Design review of the part built by this model. Coordinates are the model's own, in mm. A direction names the side the tool comes from. Round coordinates to 2 decimals unless told otherwise and drop trailing zeros. Loops run counter-clockwise (first coordinate to the right, second up) from the corner with the lowest first, then second, coordinate; pieces in that order, holes last. Notation, with made-up numbers: (85, 40.25) -> (126, 40.25) arc R17 ccw to (126, 52.25) -> close; hole circle Ø10 at (0, 55.25). An arc over 180 degrees is marked (long way). Answer as CSV lines item,"result". Start each with the question number.
```python
from build123d import *

# Parameters (mm, degrees)
F0_R     = 6.35
F1_DEPTH = 12.7


with BuildPart() as f1:
    # F0 (on Top) → F1 (new body)
    with BuildSketch(Plane.XY):
        Polygon((-7.92159, -12.359408), (-7.92159, -30.139408), (-33.32159, -30.139408), (-38.40159, -55.026224), (-7.92159, -55.026224), (-7.92159, -72.806224), (30.17841, -72.806224), (30.17841, -55.026224), (55.57841, -55.026224), (60.65841, -30.139408), (30.17841, -30.139408), (30.17841, -12.359408), align=None)
        with Locations((10.291242, -62.124663)):
            Circle(F0_R, mode=Mode.SUBTRACT)
        with Locations((-20.188758, -41.804663)):
            Circle(F0_R, mode=Mode.SUBTRACT)
        with Locations((10.291242, -41.804663)):
            Circle(F0_R, mode=Mode.SUBTRACT)
        with Locations((10.291242, -21.484663)):
            Circle(F0_R, mode=Mode.SUBTRACT)
        with Locations((40.771242, -41.804663)):
            Circle(F0_R, mode=Mode.SUBTRACT)
    extrude(amount=F1_DEPTH)


solid = f1.part
```
Q1. Mouldability with a two-part tool opening along Y and no side actions: class faces 6 (the flat face through (43, -55.026, 6)), 7 (the cylindrical face through (39.395, -48.004, 6.261)), 8 (the flat face through (30.178, -21, 6)) as pulls with the +Y half, pulls with the -Y half, needs draft (parallel to the pull), parting line crosses it, or undercut.
Q2. To check wall thickness, follow probe 1 along X at (y, z) = (-47, 11); probe 2 along X at (y, z) = (-19.5, 10.25); probe 3 along Y at (x, z) = (-17.5, 2.75). State the ranges of each line that lie inside material, in increasing order. Write a range as from..to.
Q3. Add section A-A, the plane y = -18. Give the boundary of the cut face in (x, z).
Q4. Machinability: for faces 1 (the flat face through (-7.922, -64, 6)), 2 (the flat face through (-7.922, -21, 6)), 3 (the cylindrical face through (13.22, -27.12, 6.26)), 4 (the flat face through (30.178, -64, 6)), 5 (the flat face through (46, -30.139, 6)), which of the approach directions +Z, -Z, +X, -X, +Y, -Y give a long, thin tool a straight path to every point of the face, cutting with its end or side? Answer none if there is none.
Q5. Add section D-D, the plane x = 32.5. Give the boundary of the cut face in (y, z).
Q6. For pin 1 Ø6 at (y, z) = (-48.5, 7.5) entering from -X; pin 2 Ø6.5 at (x, z) = (46, 4.5) entering from +Y; pin 3 Ø4 at (y, z) = (-25.5, 6) entering from -X, all flat-tipped, find the tip position at first contact; note any pin that passes through.
Q7. Add section B-B, the plane x = -21. Give the boundary of the cut face in (y, z).
Q8. Add section C-C, the plane z = 10.5. Give the boundary of the cut face in (x, y).
Worked answers:
1,face 6,"pulls with the -Y half"
1,face 7,"undercut"
1,face 8,"needs draft"
2,probe 1,"x = -36.76..-23.84, -16.54..6.64, 13.94..37.12, 44.42..57.22"
2,probe 2,"x = -7.92..4.26, 16.32..30.18"
2,probe 3,"y = -55.03..-47.56, -36.05..-30.14"
3,outline,"(-7.92, 0) -> (4.98, 0) -> (4.98, 12.7) -> (-7.92, 12.7) -> close; (15.6, 0) -> (30.18, 0) -> (30.18, 12.7) -> (15.6, 12.7) -> close"
4,face 1,"+Z, -Z, -X, -Y"
4,face 2,"+Z, -Z, -X, +Y"
4,face 3,"+Z, -Z"
4,face 4,"+Z, -Z, +X, -Y"
4,face 5,"+Z, -Z, +X, +Y"
5,outline,"(-55.03, 0) -> (-30.14, 0) -> (-30.14, 12.7) -> (-55.03, 12.7) -> close"
6,pin 1,"stops at x = -37.68"
6,pin 2,"stops at y = -30.14"
6,pin 3,"stops at x = -7.92"
7,outline,"(-55.03, 0) -> (-48.1, 0) -> (-48.1, 12.7) -> (-55.03, 12.7) -> close; (-35.51, 0) -> (-30.14, 0) -> (-30.14, 12.7) -> (-35.51, 12.7) -> close"
8,outline,"(-38.4, -55.03) -> (-7.92, -55.03) -> (-7.92, -72.81) -> (30.18, -72.81) -> (30.18, -55.03) -> (55.58, -55.03) -> (60.66, -30.14) -> (30.18, -30.14) -> (30.18, -12.36) -> (-7.92, -12.36) -> (-7.92, -30.14) -> (-33.32, -30.14) -> close; hole circle Ø12.7 at (-20.19, -41.8); hole circle Ø12.7 at (10.29, -62.12); hole circle Ø12.7 at (10.29, -41.8); hole circle Ø12.7 at (10.29, -21.48); hole circle Ø12.7 at (40.77, -41.8)"
